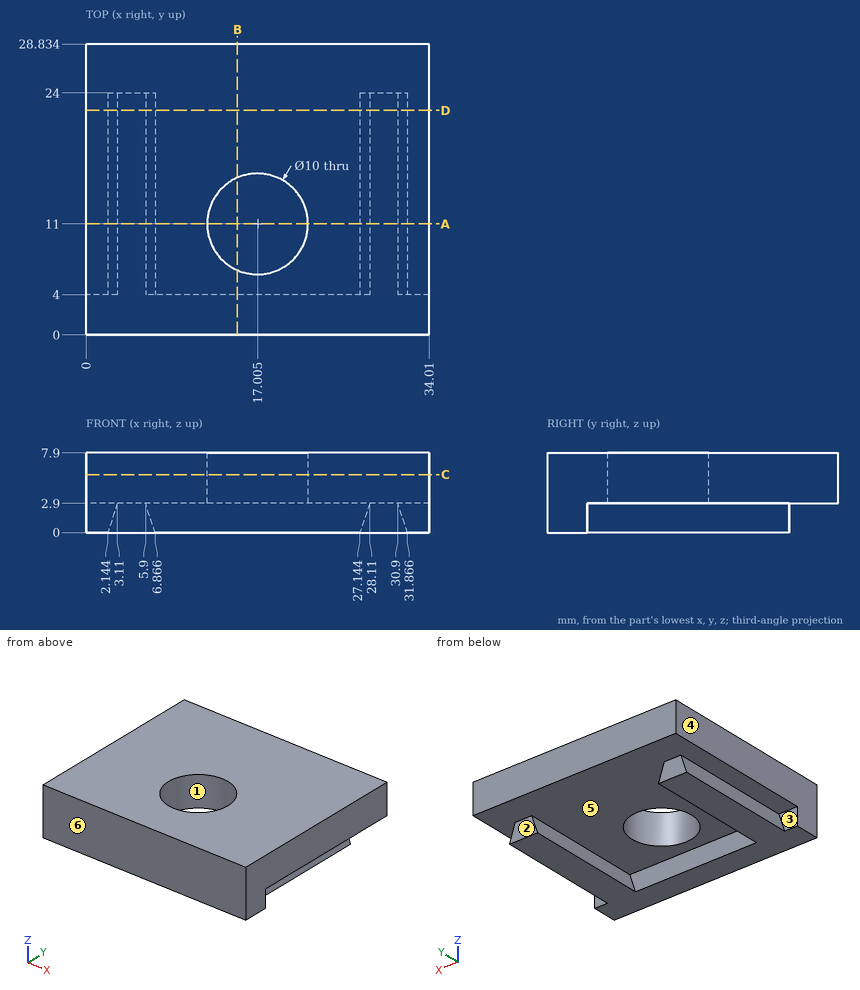
For this review, use the dimensioned drawing (mm, ordinates from the lowest corner) and the shaded views. A direction names the side the tool comes from. Give positions to 0.01 mm unless a question says otherwise; leave off trailing zeros. Order: outer loops, then holes, each group sorted by start corner. A loop starts at its lowest first (then second) coordinate and runs counter-clockwise, first axis right, second up. Notation, with made-up numbers: M -22.75,-16.5 L 22.25,-16.5 A19 ccw 22.25,-6.5 Z; hole C 15.5,-25 d5. An arc over 180 degrees is marked long. One line per question, with ' | ' between items. Start each with the question number.
1) Consider section B-B, the plane x = 15. Give the boundary of the cut face in (y, z) (1 decimal), then the cut area to 3 significant figures.
2) Consider section D-D, the plane y = 22.25. Give the boundary of the cut face in (x, z).
3) Mouldability with a two-part tool opening along X and no side actions: class the marked faces 4, 5 and 6 as pulls with the +X half, pulls with the -X half, needs draft (parallel to the pull), parting line crosses it, or undercut.
4) Consider section A-A, the plane y = 11. Give the boundary of the cut face in (x, z) (1 decimal), then the cut area to 3 significant figures.
5) Wall thickness on L1, parallel to Z at x = 8, y = 23; L2, parallel to Y at x = 30, z = 1.75; L3, parallel to Y at x = 14, z = 7.5 (1 decimal): over which ranges is each line inside the solid? List them lowest first. Write a range as from..to.
6) Consider section C-C, the plane z = 5.75. Give the boundary of the cut face in (x, y) (1 decimal), then the cut area to 3 significant figures.
7) Clearance check with flat-ended pins moving along their axes: P1, Ø12.5, axis at x = 17.5, y = 18, coming from the -Z side; P2, Ø1.5, axis at x = 4, z = 1.5, coming from the +Y side; P3, Ø12, axis at x = 8.5, y = 10, coming from the -Z side; P4, Ø8, axis at x = 17.01, y = 11, coming from the -Z side. State where each tip first meets the part, or that it passes through.
8) For the marked faces 1, 2 and 3, list the 3-axis set-ups (+Z, -Z, +X, -X, +Y, -Y) from which the entire face can be reached by the end or side of a thin tool; tool diameter is ignored.
Found:
1) outline: M 0,0 L 4,0 L 4,2.9 L 6.4,2.9 L 6.4,7.9 L 0,7.9 Z; M 15.6,2.9 L 28.8,2.9 L 28.8,7.9 L 15.6,7.9 Z | area: 110 mm²
2) outline: M 0,2.9 L 3.11,2.9 L 2.14,0 L 6.87,0 L 5.9,2.9 L 28.11,2.9 L 27.14,0 L 31.87,0 L 30.9,2.9 L 34.01,2.9 L 34.01,7.9 L 0,7.9 Z
3) face 4: pulls with the -X half | face 5: undercut | face 6: needs draft
4) outline: M 0,2.9 L 3.1,2.9 L 2.1,0 L 6.9,0 L 5.9,2.9 L 12,2.9 L 12,7.9 L 0,7.9 Z; M 22,2.9 L 28.1,2.9 L 27.1,0 L 31.9,0 L 30.9,2.9 L 34,2.9 L 34,7.9 L 22,7.9 Z | area: 142 mm²
5) L1: z = 2.9..7.9 | L2: y = 0..24 | L3: y = 0..7, 15..28.8
6) outline: M 0,0 L 34,0 L 34,28.8 L 0,28.8 Z; hole C 17,11 d10 | area: 902 mm²
7) P1: stops at z = 2.9 | P2: stops at y = 24 | P3: stops at z = 0 | P4: passes through
8) face 1: +Z, -Z | face 2: -Z, +X, -X, +Y | face 3: -X, +Y
